```python
from build123d import *

# Parameters (mm, degrees)
F1_DEPTH = 5
F2_D     = 1
F3_D     = 1


with BuildPart() as f1:
    # F0 (on Front) → F1 (new body)
    with BuildSketch(Plane.XZ):
        Polygon((-5, 20), (0, 20), (0, 40), align=None)
        Polygon((0, 20), (0, 0), (5, 20), align=None)
        Polygon((0, 40), (0, 20), (5, 20), align=None)
        Polygon((-5, 20), (0, 0), (0, 20), align=None)
    extrude(amount=F1_DEPTH)

    # F2 (through all)
    with Locations(Plane(origin=(0, 0, 0), x_dir=(1, 0, 0), z_dir=(0, 1, 0))):
        with Locations((0, -20)):
            Hole(F2_D / 2)

    # F3 (through all)
    with Locations(Plane(origin=(0, 0, 0), x_dir=(1, 0, 0), z_dir=(0, 1, 0))):
        with Locations((0, -4), (0, -36)):
            Hole(F3_D / 2)


solid = f1.part
```
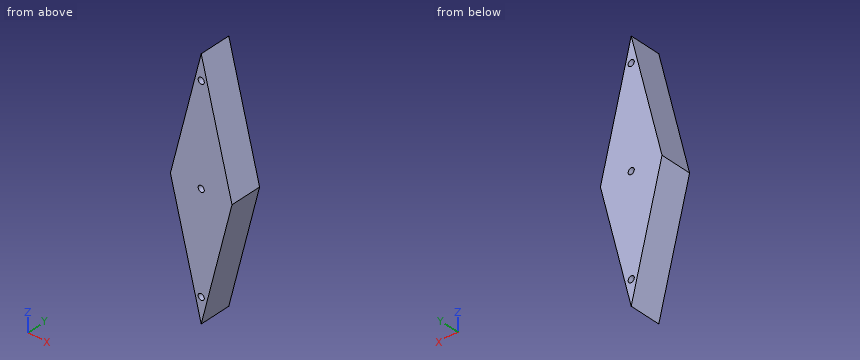
The listing builds one solid part. Answer for the finished solid, in the listing's coordinates (mm). Round coordinates to 2 decimals unless told otherwise and drop trailing zeros. Order: outer loops, then holes, each group sorted by start corner. A loop starts at its lowest first (then second) coordinate and runs counter-clockwise, first axis right, second up. Notation, with made-up numbers: (41.5, 10.5) -> (74.5, 10.5) arc R18 ccw to (74.5, 40.5) -> close; hole circle Ø6 at (45, 59). An arc over 180 degrees is marked (long way). Answer as CSV lines item,"result".
Q1. A cutting plane is placed at C-C on x = 3.25. Determine the outline of the cut face in (y, z), plus the area to 3 significant figures.
Computed values:
outline,"(-5, 13) -> (0, 13) -> (0, 27) -> (-5, 27) -> close"
area,"70.0 mm^2"
Q2. A cutting plane is placed at D-D on z = 16. Determine the outline of the cut face in (x, y).
Computed values:
outline,"(-4, -5) -> (4, -5) -> (4, 0) -> (-4, 0) -> close"
Q3. Given pin 1 (1.5 mm diameter, centred on y = -1, z = 22.5, fed in from -X); pin 2 (1 mm diameter, centred on y = -2.5, z = 24.5, fed in from -X); pin 3 (1 mm diameter, centred on y = -1.5, z = 28.5, fed in from -X), each flat-ended and moving along its own axis, determine where each tip first touches the part or whether it passes through.
Computed values:
pin 1,"stops at x = -4.56"
pin 2,"stops at x = -4"
pin 3,"stops at x = -3"
Q4. Consider line 1 (X direction, y = -3.8, z = 20); line 2 (X direction, y = -2.8, z = 36); line 3 (X direction, y = -0.35, z = 17.5) (3 decimals). Determine where each line is inside the solid, lowest interval first. Write a range as from..to.
Computed values:
line 1,"x = -5..-0.5, 0.5..5"
line 2,"x = -1..-0.5, 0.5..1"
line 3,"x = -4.375..4.375"
Q5. A cutting plane is placed at A-A on z = 36. Determine the outline of the cut face in (x, y), plus the area to 3 significant figures.
Computed values:
outline,"(-1, -5) -> (-0.5, -5) -> (-0.5, 0) -> (-1, 0) -> close; (0.5, -5) -> (1, -5) -> (1, 0) -> (0.5, 0) -> close"
area,"5.00 mm^2"
Q6. A cutting plane is placed at B-B on y = -4.15. Determine the outline of the cut face in (x, z), plus the area to 3 significant figures.
Computed values:
outline,"(-5, 20) -> (0, 0) -> (5, 20) -> (0, 40) -> close; hole circle Ø1 at (0, 4); hole circle Ø1 at (0, 20); hole circle Ø1 at (0, 36)"
area,"198 mm^2"
